The model under review builds one solid part; all positions refer to its coordinate system, in mm. A direction names the side the tool comes from. Coordinates: 2 decimals unless noted, no trailing zeros. Loops run counter-clockwise (first coordinate to the right, second up) from the corner with the lowest first, then second, coordinate; pieces in that order, holes last. Notation, with made-up numbers: M 45.25,42.25 L 97.25,42.25 A30 ccw 97.25,64.25 Z; hole C 45,42.25 d1. An arc over 180 degrees is marked long. Use CSV: the item, a comma, the result in double quotes. Start each with the question number.
from build123d import *

# Parameters (mm, degrees)
CYLINDER002_R          = 2
CYLINDER002_DEPTH      = 11
ARRAY002_X_COUNT       = 2
ARRAY002_X_PITCH       = 103
ARRAY002_Z_COUNT       = 2
ARRAY002_Z_PITCH       = 91
BOX_W                  = 8
BOX_H                  = 20
BOX_DEPTH              = 24
BOX001_W               = 8
BOX001_H               = 20
BOX001_DEPTH           = 24
BOX002_W               = 37
BOX002_H               = 7
BOX002_DEPTH           = 7
BOX003_W               = 37
BOX003_H               = 7
BOX003_DEPTH           = 7
CYLINDER_R             = 2.5
CYLINDER_DEPTH         = 20
CYLINDER_ROLL_ANGLE    = 90
ARRAY_X_COUNT          = 2
ARRAY_X_PITCH          = 73
ARRAY_Z_COUNT          = 2
ARRAY_Z_PITCH          = 80
CYLINDER001_R          = 2
CYLINDER001_DEPTH      = 20
CYLINDER001_ROLL_ANGLE = 90
ARRAY001_X_COUNT       = 2
ARRAY001_X_PITCH       = 28
ARRAY001_Z_COUNT       = 2
ARRAY001_Z_PITCH       = 50
BOX004_W               = 6.5
BOX004_H               = 16
BOX004_DEPTH           = 3.5
ARRAY003_X_COUNT       = 2
ARRAY003_X_PITCH       = 103
ARRAY003_Z_COUNT       = 2
ARRAY003_Z_PITCH       = 90.5
EXTRUDE001_DEPTH       = 100


with BuildPart() as h_bolts_union:
    # Cylinder002 → Cylinder002 (new body)
    with BuildSketch(Plane(origin=(5, 10, -1), x_dir=(1, 0, 0), z_dir=(0, 0, 1))):
        Circle(CYLINDER002_R)
    extrude(amount=CYLINDER002_DEPTH)

    # Array002 X: h_bolts_union ×2


with BuildPart() as h_bolts_union_1:
    add(h_bolts_union.part)
    with Locations(*[(i * ARRAY002_X_PITCH, 0, 0) for i in range(1, ARRAY002_X_COUNT)]):
        add(h_bolts_union.part)

    # Array002 Z: h_bolts_union ×2


with BuildPart() as h_bolts_union_2:
    add(h_bolts_union_1.part)
    with Locations(*[(0, 0, i * ARRAY002_Z_PITCH) for i in range(1, ARRAY002_Z_COUNT)]):
        add(h_bolts_union_1.part)


with BuildPart() as h_bearing_up_v:
    # Box → Box (new body)
    with BuildSketch(Plane(origin=(64.5, -5, 64), x_dir=(1, 0, 0), z_dir=(0, 0, 1))):
        with Locations((4, 10)):
            Rectangle(BOX_W, BOX_H)
    extrude(amount=BOX_DEPTH)


with BuildPart() as h_bearing_dn_v:
    # Box001 → Box001 (new body)
    with BuildSketch(Plane(origin=(64.5, -5, 13.5), x_dir=(1, 0, 0), z_dir=(0, 0, 1))):
        with Locations((4, 10)):
            Rectangle(BOX001_W, BOX001_H)
    extrude(amount=BOX001_DEPTH)


with BuildPart() as h_bearing_dn_h:
    # Box002 → Box002 (new body)
    with BuildSketch(Plane(origin=(50, -1, 22), x_dir=(1, 0, 0), z_dir=(0, 0, 1))):
        with Locations((18.5, 3.5)):
            Rectangle(BOX002_W, BOX002_H)
    extrude(amount=BOX002_DEPTH)


with BuildPart() as h_bearing_up_h:
    # Box003 → Box003 (new body)
    with BuildSketch(Plane(origin=(50, -1, 72), x_dir=(1, 0, 0), z_dir=(0, 0, 1))):
        with Locations((18.5, 3.5)):
            Rectangle(BOX003_W, BOX003_H)
    extrude(amount=BOX003_DEPTH)


with BuildPart() as h_holes_extra_arr:
    # Cylinder → Cylinder (new body)
    with BuildSketch(Plane.XY):
        Circle(CYLINDER_R)
    extrude(amount=CYLINDER_DEPTH)


with BuildPart() as h_holes_extra_arr_1:
    # Cylinder roll: moved
    add(h_holes_extra_arr.part.rotate(Axis((0, 0, 0), (1, 0, 0)), CYLINDER_ROLL_ANGLE))


with BuildPart() as h_holes_extra_arr_2:
    # Cylinder placement: moved
    add(h_holes_extra_arr_1.part.moved(Location((20, 15, 10))))

    # Array X: h_holes_extra_arr ×2


with BuildPart() as h_holes_extra_arr_3:
    add(h_holes_extra_arr_2.part)
    with Locations(*[(i * ARRAY_X_PITCH, 0, 0) for i in range(1, ARRAY_X_COUNT)]):
        add(h_holes_extra_arr_2.part)

    # Array Z: h_holes_extra_arr ×2


with BuildPart() as h_holes_extra_arr_4:
    add(h_holes_extra_arr_3.part)
    with Locations(*[(0, 0, i * ARRAY_Z_PITCH) for i in range(1, ARRAY_Z_COUNT)]):
        add(h_holes_extra_arr_3.part)


with BuildPart() as h_bearing_bolt:
    # Cylinder001 → Cylinder001 (new body)
    with BuildSketch(Plane.XY):
        Circle(CYLINDER001_R)
    extrude(amount=CYLINDER001_DEPTH)


with BuildPart() as h_bearing_bolt_1:
    # Cylinder001 roll: moved
    add(h_bearing_bolt.part.rotate(Axis((0, 0, 0), (1, 0, 0)), CYLINDER001_ROLL_ANGLE))


with BuildPart() as h_bearing_bolt_2:
    # Cylinder001 placement: moved
    add(h_bearing_bolt_1.part.moved(Location((55, 15, 25.5))))

    # Array001 X: h_bearing_bolt ×2


with BuildPart() as h_bearing_bolt_3:
    add(h_bearing_bolt_2.part)
    with Locations(*[(i * ARRAY001_X_PITCH, 0, 0) for i in range(1, ARRAY001_X_COUNT)]):
        add(h_bearing_bolt_2.part)

    # Array001 Z: h_bearing_bolt ×2


with BuildPart() as h_bearing_bolt_4:
    add(h_bearing_bolt_3.part)
    with Locations(*[(0, 0, i * ARRAY001_Z_PITCH) for i in range(1, ARRAY001_Z_COUNT)]):
        add(h_bearing_bolt_3.part)


with BuildPart() as holes:
    # Box004 → Box004 (new body)
    with BuildSketch(Plane(origin=(1.75, 5, 3), x_dir=(1, 0, 0), z_dir=(0, 0, 1))):
        with Locations((3.25, 8)):
            Rectangle(BOX004_W, BOX004_H)
    extrude(amount=BOX004_DEPTH)

    # Array003 X: holes ×2


with BuildPart() as holes_1:
    add(holes.part)
    with Locations(*[(i * ARRAY003_X_PITCH, 0, 0) for i in range(1, ARRAY003_X_COUNT)]):
        add(holes.part)

    # Array003 Z: holes ×2


with BuildPart() as holes_2:
    add(holes_1.part)
    with Locations(*[(0, 0, i * ARRAY003_Z_PITCH) for i in range(1, ARRAY003_Z_COUNT)]):
        add(holes_1.part)

    # Fusion: union h_bolts_union, h_bearing_up_v, h_bearing_dn_v, h_bearing_dn_h, h_bearing_up_h, h_holes_extra_arr, h_bearing_bolt
    add(h_bolts_union_2.part)
    add(h_bearing_up_v.part)
    add(h_bearing_dn_v.part)
    add(h_bearing_dn_h.part)
    add(h_bearing_up_h.part)
    add(h_holes_extra_arr_4.part)
    add(h_bearing_bolt_4.part)


with BuildPart() as cut:
    # Sketch → Extrude001 (new body)
    with BuildSketch(Plane.XY):
        Polygon((-56.5, 20), (-46.5, 20), (-46.5, 10), (46.5, 10), (46.5, 20), (56.5, 20), (56.5, 0), (-56.5, 0), align=None)
    extrude(amount=EXTRUDE001_DEPTH)


with BuildPart() as cut_1:
    # Extrude001 placement: moved
    add(cut.part.moved(Location((56.5, 0, 0))))

    # Cut: cut holes
    add(holes_2.part, mode=Mode.SUBTRACT)


solid = cut_1.part
1. Add section A-A (y = 13.5). Write out the cut boundary in (x, z).
2. Add section C-C (x = 67). Write out the cut boundary in (y, z), plus the area to 3 significant figures.
3. Draft analysis for pull direction X (two halves, no side actions). For faces 5 (the cylindrical face through (54.566, 8.028, 23.548)), 6 (the flat face through (57, 6, 0)), 7 (the flat face through (72.5, 7, 76)), 8 (the flat face through (0, 10, 49)), state which applies: released by +X, released by -X, zero draft, split by the parting line, or undercut.
4. Add section B-B (z = 25.5). Write out the cut boundary in (x, y).
5. Insertion check: pin 1 Ø2.5 at (x, y) = (108, 10) entering from -Z; pin 2 Ø4 at (x, z) = (107, 95) entering from +Y; pin 3 Ø3 at (x, z) = (20, 10) entering from -Y; pin 4 Ø3 at (x, y) = (5, 10) entering from +Z. Each pin has a flat end and moves straight along its axis. Give the tip position at first contact, or say it passes through.
6. Add section D-D (x = 93). Write out the cut boundary in (y, z).
7. For faces 1 (the flat face through (64.5, 7, 76)), 2 (the flat face through (57, 3, 72)), 3 (the flat face through (1.75, 12, 95)), 4 (the flat face through (5, 10, 10)), list the 3-axis set-ups (+Z, -Z, +X, -X, +Y, -Y) from which the entire face can be reached by the end or side of a thin tool; tool diameter is ignored.
8. To check wall thickness, follow line 1 along Z through (x, y) = (20, 3.5); line 2 along X through (y, z) = (8.85, 75.5); line 3 along Z through (x, y) = (54, 3.5). State the ranges of each line that lie inside material, in increasing order.
Solved:
1,outline,"M 0,0 L 10,0 L 10,100 L 0,100 Z; M 103,0 L 113,0 L 113,100 L 103,100 Z; hole M 1.75,3 L 8.25,3 L 8.25,6.5 L 1.75,6.5 Z; hole M 1.75,93.5 L 8.25,93.5 L 8.25,97 L 1.75,97 Z; hole M 104.75,3 L 111.25,3 L 111.25,6.5 L 104.75,6.5 Z; hole M 104.75,93.5 L 111.25,93.5 L 111.25,97 L 104.75,97 Z"
2,outline,"M 0,0 L 10,0 L 10,13.5 L 0,13.5 Z; M 0,37.5 L 10,37.5 L 10,64 L 0,64 Z; M 0,88 L 10,88 L 10,100 L 0,100 Z"
2,area,"520 mm^2"
3,face 5,"undercut"
3,face 6,"zero draft"
3,face 7,"undercut"
3,face 8,"released by -X"
4,outline,"M 0,0 L 50,0 L 50,6 L 53,6 L 53,10 L 10,10 L 10,20 L 0,20 Z; M 57,6 L 64.5,6 L 64.5,10 L 57,10 Z; M 72.5,6 L 81,6 L 81,10 L 72.5,10 Z; M 85,6 L 87,6 L 87,0 L 113,0 L 113,20 L 103,20 L 103,10 L 85,10 Z"
5,pin 1,"stops at z = 10"
5,pin 2,"stops at y = 20"
5,pin 3,"passes through"
5,pin 4,"stops at z = 90"
6,outline,"M 0,0 L 10,0 L 10,7.5 L 0,7.5 Z; M 0,12.5 L 10,12.5 L 10,87.5 L 0,87.5 Z; M 0,92.5 L 10,92.5 L 10,100 L 0,100 Z"
7,face 1,"+Y, -Y"
7,face 2,"-Y"
7,face 3,"+Y"
7,face 4,"-Z"
8,line 1,"z = 0 to 7.5, 12.5 to 87.5, 92.5 to 100"
8,line 2,"x = 0 to 53, 57 to 64.5, 72.5 to 81, 85 to 113"
8,line 3,"z = 0 to 22, 29 to 72, 79 to 100"
